Work out the finished part from the listing and answer in its coordinate system (mm). A direction names the side the tool comes from. Round coordinates to 2 decimals unless told otherwise and drop trailing zeros. Order: outer loops, then holes, each group sorted by start corner. A loop starts at its lowest first (then second) coordinate and runs counter-clockwise, first axis right, second up. Notation, with made-up numbers: (80, 49) - (132, 49) arc R24 cw to (132, 87) - close; hole circle Ø1 at (-28.75, 31.25). An arc over 180 degrees is marked (long way). Use one line per item in the form item = value. Start each with the question number.
Q1. Given P1, Ø9, axis at x = -19, z = -14, coming from the -Y side; P2, Ø9, axis at y = 30, z = -50, coming from the -X side; P3, Ø12, axis at y = 34.5, z = -47, coming from the -X side; P4, Ø10, axis at y = 21, z = -33.5, coming from the +X side, each flat-ended and moving along its own axis, determine where each tip first touches the part or whether it passes through.
Q2. The part is cut by section C-C on x = -19. Determine the outline of the cut face in (y, z), plus the area to 3 significant figures.
Q3. The part is cut by section B-B on y = 30. Determine the outline of the cut face in (x, z).
Q4. For a pull along Y with two mould halves and no side action, classify faces 1 (the cylindrical face through (25.303, 15.264, -8.874)), 2 (the cylindrical face through (62.994, 24.45, -8.874)), 3 (the cylindrical face through (-17.37, 5.07, -93.32)) as +Y half, -Y half, draft (parallel to the pull), parting line (faces both ways), or undercut.
Q5. Which of the six approach directions +Z, -Z, +X, -X, +Y, -Y give full straight-line access (tool end or side, diameter ignored) to faces 4 (the cylindrical face through (5, 34, -47)), 5 (the flat face through (-19, 10, -49)), 6 (the cylindrical face through (11.52, 24.65, -19.43))?
Q6. The part is cut by section D-D on z = -50. Determine the outline of the cut face in (x, y).
Q7. The part is cut by section A-A on z = -14. Determine the outline of the cut face in (x, y), plus the area to 3 significant figures.
Q8. Find the intervals of material crossed by line 1 (Z direction, x = -19, y = 6.25); line 2 (Z direction, x = 33.5, y = 3.5); line 3 (X direction, y = 39.5, z = -49), in increasing order. Write a range as [from, to].
Autodesk Fusion 360 part; units mm, degrees
sketch "Sketch1" plane through (0, 0, 0) normal (0, 0, 1) x (1, 0, 0)
  line L0 (0, 0) -> (38, 0)
  line L1 (38, 0) -> (38, 50)
  line L2 (38, 50) -> (0, 50)
  line L3 (0, 50) -> (0, 0)
  circle A0 centre (38, 25) radius 25
  circle A1 centre (38, 25) radius 16
  dimension "d1" = 38
  dimension "d2" = 50
  dimension "d3" = 50
  dimension "d5" = 32
extrude "Extrude1" add sketch "Sketch1" against normal blind 100 contours L0 L2 L3 A0 | L1 A0 A1 | L1 A0 A1
sketch "Sketch2" plane through (0, 0, 0) normal (0, -1, 0) x (1, 0, 0)
  line L0 (38, 0) -> (0, 0)
  line L1 (0, 0) -> (0, -100) construction
  line L2 (0, -100) -> (38, -100)
  line L3 (38, -100) -> (38, 0)
  line L4 (0, -50) -> (10, -50) construction
  line L5 (10, -50) -> (10, -18)
  line L6 (10, -50) -> (10, -82)
  dimension "d8" = 32
  dimension "d9" = 32
sketch "Sketch3" plane through (0, 0, 0) normal (0, -1, 0) x (1, 0, 0)
  line L0 (38, 0) -> (0, 0)
  line L1 (0, 0) -> (0, -100)
  line L2 (0, -100) -> (38, -100)
  line L3 (38, -100) -> (38, 0)
ref_plane "WorkPlane1" through (31.5, 25, -50) normal (0, 0, -1) x (-1, 0, 0)
sketch "Sketch4" plane through (31.5, 25, -50) normal (0, 0, -1) x (1, 0, 0)
sketch "Sketch5" plane through (0, 0, 0) normal (0, 0, 1) x (-1, 0, 0)
  circle A0 centre (-38, -25) radius 16
  arc A1 (-38, 0) -> (-38, -50) centre (-38, -25) ccw
  line L0 (-38, -50) -> (0, -50)
  line L1 (0, -50) -> (0, 0)
  line L2 (0, 0) -> (-38, 0)
  line L3 (0, 0) -> (38, 0)
  line L4 (38, 0) -> (38, -10)
  line L5 (38, -10) -> (0, -10)
  line L6 (0, -10) -> (0, 0)
  dimension "d10" = 38
  dimension "d11" = 10
extrude "Extrude2" add sketch "Sketch5" against normal blind 100 contours L1 L3 L4 L5 L6
sketch "Sketch6" plane through (0, 10, 0) normal (0, 1, 0) x (-1, 0, 0)
  line L0 (38, 0) -> (0, 0)
  line L1 (0, 0) -> (0, -100)
  line L2 (0, -100) -> (38, -100)
  line L3 (38, -100) -> (38, 0)
  line L4 (19, 0) -> (19, -86) construction
  circle A0 centre (19, -86) radius 7.5
  line L5 (19, 0) -> (33, 0) construction
  line L6 (33, 0) -> (33, -14) construction
  line L7 (33, -14) -> (19, -14) construction
  circle A1 centre (19, -14) radius 7.5
  dimension "d14" = 86
  dimension "d15" = 15
  dimension "d16" = 14
  dimension "d17" = 14
  dimension "d18" = 15
extrude "Extrude3" cut sketch "Sketch6" against normal blind 10 contours A0 | A1
fillet "Fillet1" radius 10 1 edges at (-38, 5, 0)
fillet "Fillet2" radius 10 1 edges at (-38, 5, -100)
ref_plane "WorkPlane2" through (17.5, 25, -50) normal (0, 0, 1) x (1, 0, 0)
sketch "Sketch7" plane through (17.5, 25, -50) normal (0, 0, 1) x (1, 0, 0)
  line L0 (-17.4789, 13.5699) -> (-7.4789, 13.5699) construction
  line L1 (-7.4789, 25.0534) -> (-7.4789, -25)
  line L2 (-7.4789, 25.0534) -> (50, 25.0534)
  line L3 (50, 25.0534) -> (50, -25)
  line L4 (50, -25) -> (-7.4789, -25)
  dimension "d25" = 10
extrude "Extrude4" cut sketch "Sketch7" along normal mid plane 64
sketch "Sketch8" plane through (0, 0, 0) normal (-1, 0, 0) x (0, -1, 0)
  line L0 (-10, -100) -> (-10, 0)
  line L1 (-10, 0) -> (-50, 0)
  line L2 (-50, 0) -> (-50, -100)
  line L3 (-50, -100) -> (-10, -100)
  line L4 (-50, -50) -> (-10, -50) construction
  circle A0 centre (-30, -50) radius 5
  dimension "d28" = 10
fillet "Fillet3" radius 5 1 edges at (10.0211, 25, -18)
fillet "Fillet4" radius 5 1 edges at (10.0211, 25, -82)
extrude "Extrude5" cut sketch "Sketch8" against normal blind 10 contours A0
Found:
q1.P1 = through
q1.P2 = 10
q1.P3 = 0
q1.P4 = 10.02
q2.outline = (0, -100) - (10, -100) - (10, -93.5) - (0, -93.5) - close; (0, -78.5) - (10, -78.5) - (10, -21.5) - (0, -21.5) - close; (0, -6.5) - (10, -6.5) - (10, 0) - (0, 0) - close
q2.area = 700 mm²
q3.outline = (0, -100) - (22.8, -100) - (22.8, -82) - (15.02, -82) arc R5 cw to (10.02, -77) - (10.02, -23) arc R5 cw to (15.02, -18) - (22.8, -18) - (22.8, 0) - (0, 0) - (0, -45) - (10, -45) - (10, -55) - (0, -55) - close; (53.2, -100) - (62.49, -100) - (62.49, -82) - (53.2, -82) - close; (53.2, -18) - (62.49, -18) - (62.49, 0) - (53.2, 0) - close
q4.face_1 = undercut
q4.face_2 = parting line
q4.face_3 = draft
q5.face_4 = -X
q5.face_5 = +Z, -Z, -X, +Y
q5.face_6 = +X, +Y, -Y
q6.outline = (-38, 0) - (10.02, 0) - (10.02, 50) - (0, 50) - (0, 35) - (10, 35) - (10, 25) - (0, 25) - (0, 10) - (-38, 10) - close
q7.outline = (-38, 0) - (-26.5, 0) - (-26.5, 10) - (-38, 10) - close; (-11.5, 0) - (38, 0) arc R25 ccw to (38, 50) - (0, 50) - (0, 10) - (-11.5, 10) - close; hole circle Ø32 at (38, 25)
q7.area = 2,310 mm²
q8.line_1 = [-100, -93.5], [-78.5, -21.5], [-6.5, 0]
q8.line_2 = [-100, -82], [-18, 0]
q8.line_3 = [0, 10.02]
